Read the model definition and answer for the solid it produces. Units are mm, in the model's axes. A direction names the side the tool comes from. Round coordinates to 2 decimals unless told otherwise and drop trailing zeros. Order: outer loops, then holes, each group sorted by start corner. A loop starts at its lowest first (then second) coordinate and runs counter-clockwise, first axis right, second up. Notation, with made-up numbers: (45.5, 11.25) -> (82.5, 11.25) arc R12 cw to (82.5, 22.25) -> close; hole circle Ø7 at (59.25, 73). An arc over 180 degrees is marked (long way). One line per item, written item: value. Start each with the question number.
1. Section A-A (x = 0) is taken. Give the vertices of the cut face in (y, z).
2. Section D-D (z = 15) is taken. Give the vertices of the cut face in (x, y), then the cut area to 3 significant figures.
3. Flat-ended cylindrical pins translate along their axes: pin 1 Ø10 at (y, z) = (-7.5, 9) entering from +X; pin 2 Ø2 at (y, z) = (-8, 22.5) entering from -X; pin 3 Ø6 at (x, y) = (4, -0.5) entering from +Z. Find the tip coordinate at first contact, or state that the pin passes through.
4. Consider line 1 (Y direction, x = 0, z = 10.5); line 2 (Y direction, x = 0, z = 3.3); line 3 (Z direction, x = 6, y = 4.25). Determine where each line is inside the solid, lowest interval first.
5. Section C-C (x = -7.5) is taken. Give the vertices of the cut face in (y, z), then the cut area to 3 significant figures.
6. The mould has two halves that part along Y. Classify faces 1 (the face through (0, 8.2, 25)), 2 (the face through (-1.73, -7.81, 15.14)), 3 (the face through (-2.17, -9.76, 12.32)): released by +Y, released by -Y, zero draft, split by the parting line, or undercut.
7. For faces 4 (the face through (-4, -2, 5)), 5 (the face through (-0.1, -4.3, 0)), determine the directions among +Z, -Z, +X, -X, +Y, -Y from which every point of the face is accessible in a straight line to the end or side of a thin tool.
from build123d import *

# Parameters (mm, degrees)
F0_R     = 10
F0_R_2   = 4
F1_DEPTH = 25
F2_R     = 8
F3_DEPTH = 20
F4_DEPTH = 5


with BuildPart() as f1:
    # F0 (on Top) → F1 (new body)
    with BuildSketch(Plane.XY):
        Circle(F0_R)
        Circle(F0_R_2, mode=Mode.SUBTRACT)
    extrude(amount=F1_DEPTH)

    # F2 (on face) → F3 (cut)
    with BuildSketch(Plane.XY.offset(25)):
        Circle(F2_R)
    extrude(amount=-F3_DEPTH, mode=Mode.SUBTRACT)

    # F0 (on Top) → F4 (join)
    with BuildSketch(Plane.XY):
        Circle(F0_R)
        Circle(F0_R_2, mode=Mode.SUBTRACT)
    extrude(amount=F4_DEPTH)


solid = f1.part
Answer:
1. outline: (-10, 0) -> (-4, 0) -> (-4, 5) -> (-8, 5) -> (-8, 25) -> (-10, 25) -> close; (4, 0) -> (10, 0) -> (10, 25) -> (8, 25) -> (8, 5) -> (4, 5) -> close
2. outline: circle Ø20 at (0, 0); hole circle Ø16 at (0, 0)
2. area: 113 mm^2
3. pin 1: x = 9.68
3. pin 2: x = -7.14
3. pin 3: z = 5
4. line 1: -10 to -8, 8 to 10
4. line 2: -10 to -4, 4 to 10
4. line 3: 0 to 5
5. outline: (-6.61, 0) -> (6.61, 0) -> (6.61, 25) -> (2.78, 25) -> (2.78, 5) -> (-2.78, 5) -> (-2.78, 25) -> (-6.61, 25) -> close
5. area: 219 mm^2
6. face 1: zero draft
6. face 2: undercut
6. face 3: split by the parting line
7. face 4: +Z
7. face 5: -Z, +X, -X, +Y, -Y
